The figure shows three views and two pictorial views of one solid part (mm, origin at its lowest corner). Answer the questions. A direction names the side the tool comes from. Coordinates: 2 decimals unless noted, no trailing zeros. Order: outer loops, then holes, each group sorted by start corner. A loop starts at its lowest first (then second) coordinate and runs counter-clockwise, first axis right, second up. Notation, with made-up numbers: (-13.5, 67.25) -> (5.5, 67.25) arc R36 ccw to (5.5, 103.25) -> close; hole circle Ø9 at (12, -22.75). An arc over 180 degrees is marked (long way). Return JSON: item names as keys, results as strings.
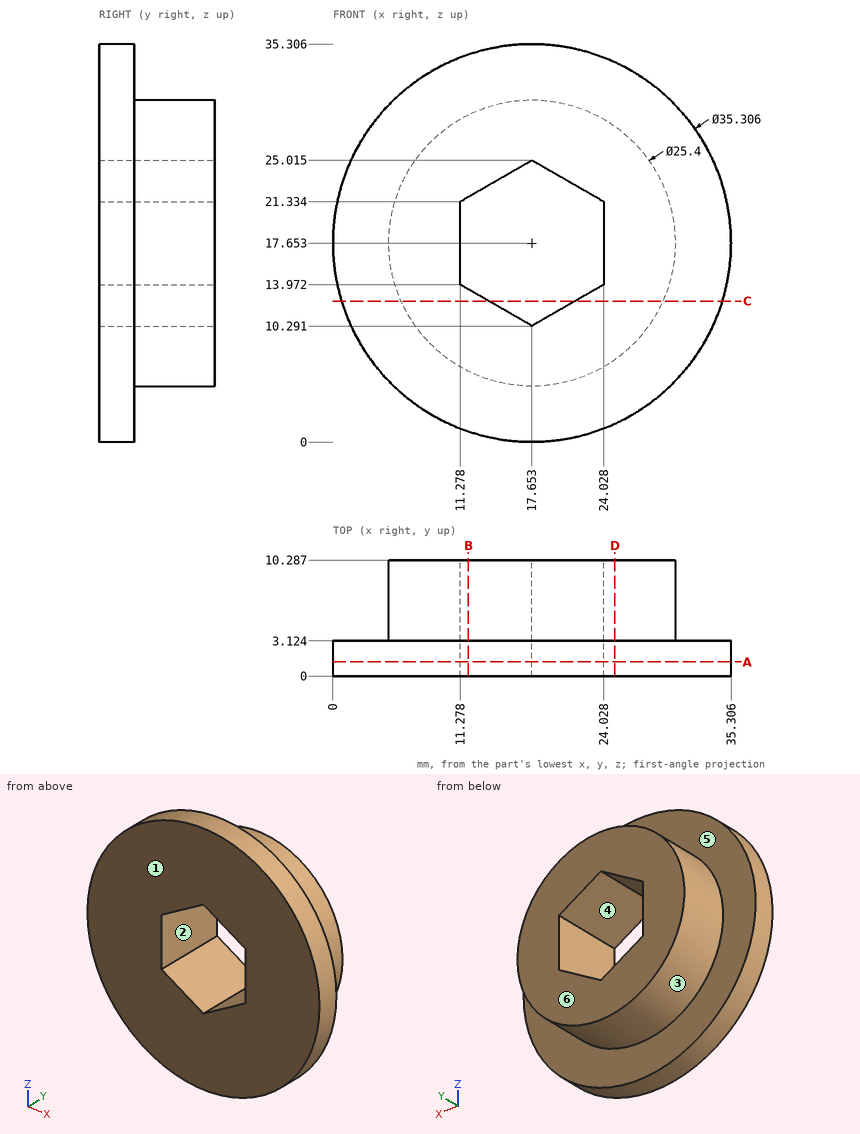
Item 1: Flat-ended cylindrical pins translate along their axes: pin 1 (5 mm diameter, centred on y = 5, z = 25, fed in from -X); pin 2 (2 mm diameter, centred on y = 7.5, z = 6.5, fed in from -X) (1 decimal); pin 3 (5 mm diameter, centred on x = 30.5, y = 3, fed in from +Z) (1 decimal). Find the tip coordinate at first contact, or state that the pin passes through.
Answer list:
{"pin 1": "x = 0.94", "pin 2": "x = 10", "pin 3": "z = 32"}
Item 2: The part is cut by section D-D on x = 25. Determine the outline of the cut face in (y, z) (1 decimal).
Answer list:
{"outline": "(0, 1.6) -> (3.1, 1.6) -> (3.1, 7.3) -> (10.3, 7.3) -> (10.3, 28) -> (3.1, 28) -> (3.1, 33.7) -> (0, 33.7) -> close"}
Item 3: The part is cut by section A-A on y = 1.25. Determine the outline of the cut face in (x, z) (1 decimal).
Answer list:
{"outline": "circle Ø35.3 at (17.7, 17.7); hole (11.3, 14) -> (17.7, 10.3) -> (24, 14) -> (24, 21.3) -> (17.7, 25) -> (11.3, 21.3) -> close"}
Item 4: The part is cut by section B-B on x = 12. Determine the outline of the cut face in (y, z) (1 decimal), plus the area to 3 significant figures.
Answer list:
{"outline": "(0, 0.9) -> (3.1, 0.9) -> (3.1, 6.3) -> (10.3, 6.3) -> (10.3, 13.6) -> (0, 13.6) -> close; (0, 21.8) -> (10.3, 21.8) -> (10.3, 29) -> (3.1, 29) -> (3.1, 34.4) -> (0, 34.4) -> close", "area": "183 mm2"}
Item 5: Determine the mould class of the marked faces 1, 2 and 3 for opening direction Z: pulls with the +Z half, pulls with the -Z half, needs draft (parallel to the pull), parting line crosses it, or undercut.
Answer list:
{"face 1": "needs draft", "face 2": "undercut", "face 3": "parting line crosses it"}
Item 6: Which of the six approach directions +Z, -Z, +X, -X, +Y, -Y give full straight-line access (tool end or side, diameter ignored) to the marked faces 4, 5 and 6?
Answer list:
{"face 4": "+Y, -Y", "face 5": "+Y", "face 6": "+Z, -Z, +X, -X, +Y"}
Item 7: The part is cut by section C-C on z = 12.5. Determine the outline of the cut face in (x, y) (1 decimal), plus the area to 3 significant figures.
Answer list:
{"outline": "(0.8, 0) -> (13.8, 0) -> (13.8, 10.3) -> (6, 10.3) -> (6, 3.1) -> (0.8, 3.1) -> close; (21.5, 0) -> (34.5, 0) -> (34.5, 3.1) -> (29.3, 3.1) -> (29.3, 10.3) -> (21.5, 10.3) -> close", "area": "193 mm2"}
Item 8: Find the intervals of material crossed by probe 1 along Y at (x, z) = (2.5, 25.5) (1 decimal); probe 2 along X at (y, z) = (5.5, 16) (1 decimal); probe 3 along X at (y, z) = (2.25, 18.5) (1 decimal), in increasing order.
Answer list:
{"probe 1": "0 to 3.1", "probe 2": "5.1 to 11.3, 24 to 30.2", "probe 3": "0 to 11.3, 24 to 35.3"}
